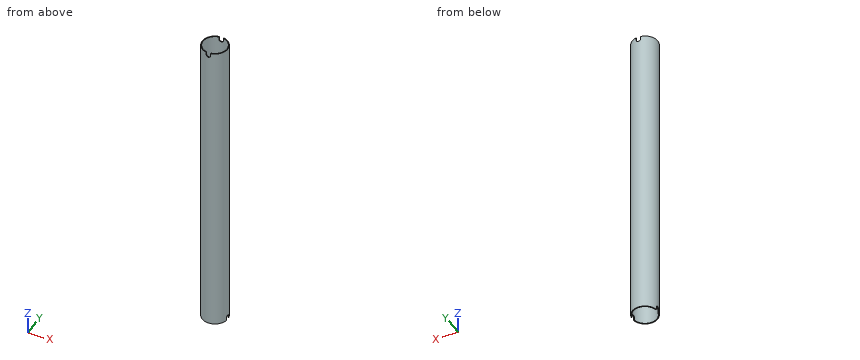
from build123d import *

# Parameters (mm, degrees)
SKETCH1_W          = 300.0375
SKETCH1_H          = 0.889
CUT_EXTRUDE1_DEPTH = 12.7
CUT_EXTRUDE2_DEPTH = 12.7
SCALE1_SCALE       = 0.6


with BuildPart() as part:
    # Sketch1 → Revolve1 (revolve)
    with BuildSketch(Plane(origin=(0, 0, 0), x_dir=(0, 0, -1), z_dir=(1, 0, 0)), mode=Mode.PRIVATE) as revolve1_sk:
        with Locations((0, 12.0015)):
            Rectangle(SKETCH1_W, SKETCH1_H)
    revolve(revolve1_sk.sketch.rotate(Axis((0, 0, 90.675886036), (0, 0, -1)), 90), axis=Axis((0, 0, 90.675886036), (0, 0, -1)))

    # Sketch2 → Cut-Extrude1 (cut, symmetric)
    with BuildSketch(Plane(origin=(0, 0, 0), x_dir=(1, 0, 0), z_dir=(0, 1, 0))):
        with BuildLine():
            Line((-2.159, -155.09875), (-2.159, -147.47875))
            ThreePointArc((-2.159, -147.47875), (0, -145.31975), (2.159, -147.47875))
            Line((2.159, -147.47875), (2.159, -155.09875))
            ThreePointArc((2.159, -155.09875), (0, -157.25775), (-2.159, -155.09875))
        make_face()
    extrude(amount=CUT_EXTRUDE1_DEPTH, both=True, mode=Mode.SUBTRACT)

    # Sketch3 → Cut-Extrude2 (cut, symmetric)
    with BuildSketch(Plane(origin=(0, 0, 0), x_dir=(0, 0, -1), z_dir=(1, 0, 0))):
        with BuildLine():
            Line((155.09875, -2.159), (147.47875, -2.159))
            ThreePointArc((147.47875, -2.159), (145.31975, 0), (147.47875, 2.159))
            Line((147.47875, 2.159), (155.09875, 2.159))
            ThreePointArc((155.09875, 2.159), (157.25775, 0), (155.09875, -2.159))
        make_face()
    extrude(amount=CUT_EXTRUDE2_DEPTH, both=True, mode=Mode.SUBTRACT)


with BuildPart() as part_1:
    # Scale1: scaled about (-1.267e-06, -7.59e-07, -4.795e-06)
    add(part.part.scale(SCALE1_SCALE).moved(Location((-5.07e-07, -3.04e-07, -1.918e-06))))


solid = part_1.part
Check sheet for the modelled part. Datum: model origin and axes. Units: mm. Round coordinates to 2 decimals unless told otherwise and drop trailing zeros. Loops run counter-clockwise (first coordinate to the right, second up) from the corner with the lowest first, then second, coordinate; pieces in that order, holes last. Notation, with made-up numbers: (0, 29.5) -> (55, 29.5) arc R18 cw to (55, 57.5) -> close; hole circle Ø8 at (36, 62). An arc over 180 degrees is marked (long way). Put each result on its own line as item: value. Start each with the question number.
1. Section check A-A (x = -3). Enter the section's corners in (y, z).
2. Gauge pin test, flat ends, axial feed: pin 1 (1 mm diameter, centred on x = -3, z = -65, fed in from -Y); pin 2 (0.6 mm diameter, centred on y = 7, z = 89, fed in from +X); pin 3 (1.5 mm diameter, centred on y = -1, z = 11.5, fed in from -X). Record the tip position at first contact, or that the pin passes through.
3. Section check C-C (z = -68). Enter the section's corners in (x, y).
4. Scan lines: probe 1 along X at (y, z) = (0, 49.5); probe 2 along X at (y, z) = (2.25, -70). Record each from-to range of solid material in increasing order.
Findings:
1. outline: (-6.84, -90.01) -> (-6.25, -90.01) -> (-6.25, 90.01) -> (-6.84, 90.01) -> close; (6.25, -90.01) -> (6.84, -90.01) -> (6.84, 90.01) -> (6.25, 90.01) -> close
2. pin 1: stops at y = -7.04
2. pin 2: stops at x = 3.3
2. pin 3: stops at x = -7.46
3. outline: circle Ø14.94 at (0, 0); hole circle Ø13.87 at (0, 0)
4. probe 1: x = -7.47 to -6.93, 6.93 to 7.47
4. probe 2: x = -7.12 to -6.56, 6.56 to 7.12
